Print and shaded views of the part. All mm, measured from the part's lowest x, y and z. Give positions to 0.01 mm unless a question says otherwise; leave off trailing zeros. Loops run counter-clockwise (first coordinate to the right, second up) from the corner with the lowest first, then second, coordinate; pieces in that order, holes last.
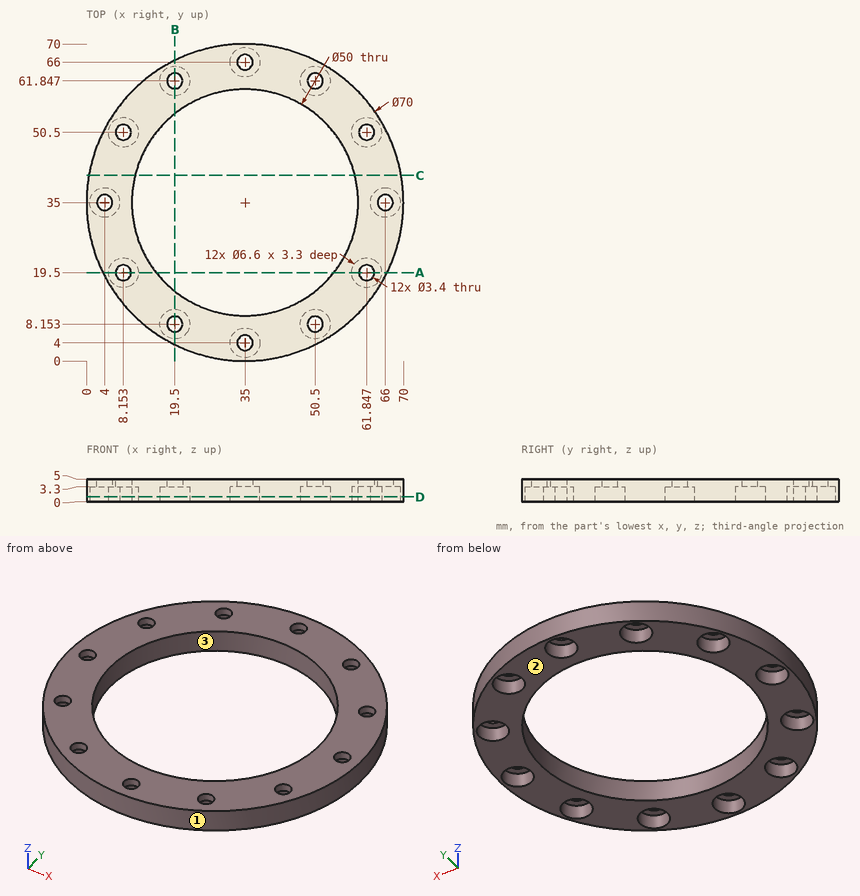
1. Probe line 1 along Y through (x, z) = (35, 3.9); line 2 along Y through (x, z) = (35, 1.4); line 3 along Y through (x, z) = (9, 0.7). List the from-to ranges inside material, lowest first.
Responses:
line 1: y = 0 to 2.3, 5.7 to 10, 60 to 64.3, 67.7 to 70
line 2: y = 0 to 0.7, 7.3 to 10, 60 to 62.7, 69.3 to 70
line 3: y = 11.57 to 16.31, 22.69 to 47.31, 53.69 to 58.43
2. Pull direction X, two halves, no side cores. Call the marked faces 1, 2 and 3: released by +X, released by -X, zero draft, split by the parting line, or undercut.
Responses:
face 1: split by the parting line
face 2: zero draft
face 3: undercut
3. Saw through at C-C, the plane y = 41. List the corners of the cut face in (x, z), and give its area (3 significant figures).
Responses:
outline: (0.52, 0) - (10.73, 0) - (10.73, 5) - (0.52, 5) - close; (59.27, 0) - (69.48, 0) - (69.48, 5) - (59.27, 5) - close
area: 102 mm2
4. Saw through at D-D, the plane z = 1.05. Count the separate pieces of the cut face and the enclosed holes in it, and give its area (3 significant figures).
Responses:
separate pieces: 1
enclosed holes: 13
area: 1,470 mm2
5. Drop flat-ended pins along their axis: pin 1 (5.5 mm diameter, centred on x = 35, y = 4, fed in from -Z); pin 2 (1.5 mm diameter, centred on y = 37, z = 3, fed in from -X); pin 3 (3 mm diameter, centred on x = 62.5, z = 1, fed in from -Y). Give the stop position or say it passes through.
Responses:
pin 1: stops at z = 3.3
pin 2: stops at x = 0.02
pin 3: stops at y = 11.57
6. Saw through at A-A, the plane y = 19.5. List the corners of the cut face in (x, z) (1 decimal).
Responses:
outline: (3.6, 0) - (4.9, 0) - (4.9, 3.3) - (6.5, 3.3) - (6.5, 5) - (3.6, 5) - close; (9.9, 3.3) - (11.5, 3.3) - (11.5, 0) - (15.4, 0) - (15.4, 5) - (9.9, 5) - close; (54.6, 0) - (58.5, 0) - (58.5, 3.3) - (60.1, 3.3) - (60.1, 5) - (54.6, 5) - close; (63.5, 3.3) - (65.1, 3.3) - (65.1, 0) - (66.4, 0) - (66.4, 5) - (63.5, 5) - close
